Read the model definition and answer for the solid it produces. Units are mm, in the model's axes. Coordinates: 2 decimals unless noted, no trailing zeros. Order: outer loops, then holes, each group sorted by start corner. A loop starts at its lowest first (then second) coordinate and runs counter-clockwise, first axis right, second up. Notation, with made-up numbers: M 36,89 L 70,89 A5 ccw 70,97 Z; hole C 25.5,74 d7. An arc over 180 degrees is marked long. One line per question, with ' | ' between items. Start each with the question number.
1) Find section C-C, the plane y = 0.4. Count the separate pieces of the cut face and the enclosed holes in it, plus the area to 3 significant figures.
2) Consider probe 1 along Z at (x, y) = (-4, 0.25); probe 2 along X at (y, z) = (0.2, 4.5); probe 3 along X at (y, z) = (0.35, 1.5). Determine where each line is inside the solid, lowest interval first.
3) Given P1, Ø6, axis at x = 1.5, z = -8, coming from the -Y side, flat-ended and moving along its own axis, determine where the tip first touches the part or whether it passes through.
4) Find section A-A, the plane x = 2.25. Write down the section's boundary in (y, z).
5) Find section B-B, the plane z = 5.75. Write down the section's boundary in (x, y), plus the area to 3 significant figures.
6) Find section D-D, the plane x = 5.75. Write down the section's boundary in (y, z).
from build123d import *

# Parameters (mm, degrees)
SKETCH1_R      = 0.25
SKETCH1_W      = 0.8
SKETCH1_H      = 2
EXTRUDE1_DEPTH = 0.5
SKETCH2_R      = 0.25
EXTRUDE2_DEPTH = 1.5


with BuildPart() as part:
    # Sketch1 → Extrude1 (new body)
    with BuildSketch(Plane(origin=(0, 0, 0), x_dir=(1, 0, 0), z_dir=(0, 1, 0))):
        Polygon((-7.071067812, 7.071067812), (0, 10), (7.071067812, 7.071067812), (10, 0), (7.071067812, -7.071067812), (0, -10), (-7.071067812, -7.071067812), (-10, 0), align=None)
        with Locations((-4, 4.5)):
            Circle(SKETCH1_R, mode=Mode.SUBTRACT)
        with Locations((4, 4.5)):
            Circle(SKETCH1_R, mode=Mode.SUBTRACT)
        with Locations((4, -4.5)):
            Circle(SKETCH1_R, mode=Mode.SUBTRACT)
        with Locations((-4, -4.5)):
            Circle(SKETCH1_R, mode=Mode.SUBTRACT)
        with Locations((0, 6)):
            Rectangle(SKETCH1_W, SKETCH1_H, mode=Mode.SUBTRACT)
        with Locations((0, -6)):
            Rectangle(SKETCH1_W, SKETCH1_H, mode=Mode.SUBTRACT)
    extrude(amount=EXTRUDE1_DEPTH)

    # Sketch2 → Extrude2 (cut, through all)
    with BuildSketch(Plane(origin=(0, 0, 0), x_dir=(1, 0, 0), z_dir=(0, 1, 0))):
        with Locations((4, 1.5)):
            Circle(SKETCH2_R)
        with Locations((4, -1.5)):
            Circle(SKETCH2_R)
        with Locations((-4, 1.5)):
            Circle(SKETCH2_R)
        with Locations((-4, -1.5)):
            Circle(SKETCH2_R)
        Polygon((3.75, 0.75), (4.25, 0.75), (4.25, 0.375), (4.5, 0.375), (4.5, -0.375), (4.25, -0.375), (4.25, -0.75), (3.75, -0.75), (3.75, -0.375), (3.5, -0.375), (3.5, 0.375), (3.75, 0.375), align=None)
        Polygon((-3.5, 0.375), (-3.5, -0.375), (-3.75, -0.375), (-3.75, -0.75), (-4.25, -0.75), (-4.25, -0.375), (-4.5, -0.375), (-4.5, 0.375), (-4.25, 0.375), (-4.25, 0.75), (-3.75, 0.75), (-3.75, 0.375), align=None)
        with BuildLine():
            Line((-6.5, 0.5), (-6.5, -0.5))
            ThreePointArc((-6.5, -0.5), (-7, 0), (-6.5, 0.5))
        make_face()
        with BuildLine():
            Line((6.5, 0.5), (6.5, -0.5))
            ThreePointArc((6.5, -0.5), (7, 0), (6.5, 0.5))
        make_face()
        with BuildLine():
            Line((-6.25, 2.75), (-5.25, 2.75))
            ThreePointArc((-5.25, 2.75), (-5.75, 2.25), (-6.25, 2.75))
        make_face()
        with BuildLine():
            Line((-2.75, 2.75), (-1.75, 2.75))
            ThreePointArc((-1.75, 2.75), (-2.25, 2.25), (-2.75, 2.75))
        make_face()
        with BuildLine():
            Line((1.75, 2.75), (2.75, 2.75))
            ThreePointArc((2.75, 2.75), (2.25, 2.25), (1.75, 2.75))
        make_face()
        with BuildLine():
            Line((5.25, 2.75), (6.25, 2.75))
            ThreePointArc((6.25, 2.75), (5.75, 2.25), (5.25, 2.75))
        make_face()
        with BuildLine():
            Line((-6.25, -2.75), (-5.25, -2.75))
            ThreePointArc((-5.25, -2.75), (-5.75, -2.25), (-6.25, -2.75))
        make_face()
        with BuildLine():
            Line((-2.75, -2.75), (-1.75, -2.75))
            ThreePointArc((-1.75, -2.75), (-2.25, -2.25), (-2.75, -2.75))
        make_face()
        with BuildLine():
            Line((1.75, -2.75), (2.75, -2.75))
            ThreePointArc((2.75, -2.75), (2.25, -2.25), (1.75, -2.75))
        make_face()
        with BuildLine():
            Line((5.25, -2.75), (6.25, -2.75))
            ThreePointArc((6.25, -2.75), (5.75, -2.25), (5.25, -2.75))
        make_face()
    extrude(amount=EXTRUDE2_DEPTH, mode=Mode.SUBTRACT)


solid = part.part
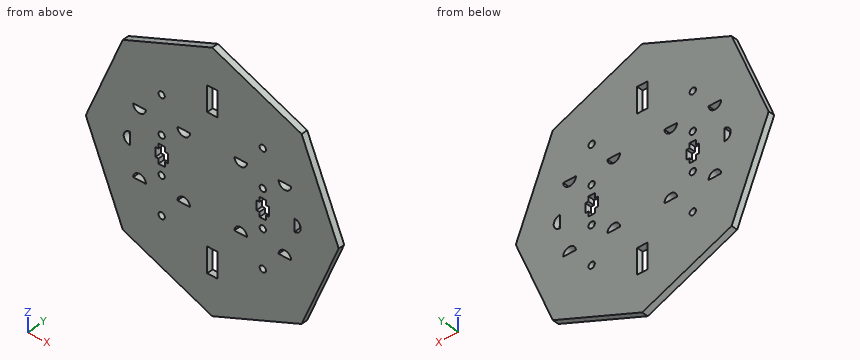
Report:
1) separate pieces: 1 | enclosed holes: 22 | area: 272 mm^2
2) probe 1: z = -8.34 to -4.75, -4.25 to -1.75, -1.25 to -0.75, 0.75 to 1.25, 1.75 to 4.25, 4.75 to 8.34 | probe 2: x = -8.14 to -4.25, -3.75 to 3.75, 4.25 to 8.14 | probe 3: x = -9.38 to -4.25, -3.75 to 3.75, 4.25 to 9.38
3) P1: stops at y = 0
4) outline: M 0,-9.07 L 0.5,-9.07 L 0.5,-2.75 L 0,-2.75 Z; M 0,-2.25 L 0.5,-2.25 L 0.5,2.25 L 0,2.25 Z; M 0,2.75 L 0.5,2.75 L 0.5,9.07 L 0,9.07 Z
5) outline: M -7.62,0 L -0.4,0 L -0.4,0.5 L -7.62,0.5 Z; M 0.4,0 L 7.62,0 L 7.62,0.5 L 0.4,0.5 Z | area: 7.22 mm^2
6) outline: M 0,-7.62 L 0.5,-7.62 L 0.5,-2.75 L 0,-2.75 Z; M 0,-2.25 L 0.5,-2.25 L 0.5,2.25 L 0,2.25 Z; M 0,2.75 L 0.5,2.75 L 0.5,7.62 L 0,7.62 Z
